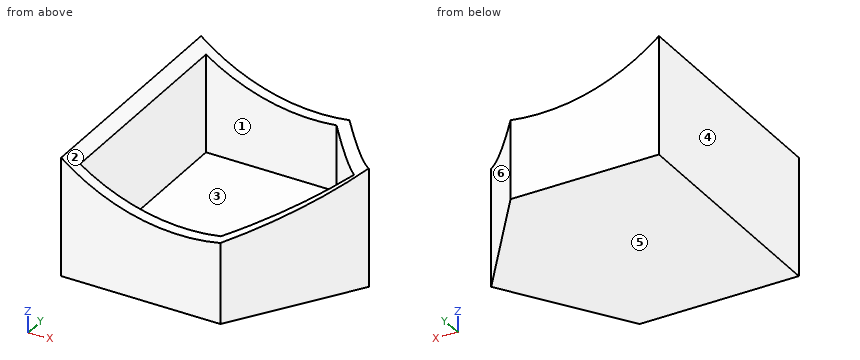
from build123d import *

# Parameters (mm, degrees)
F1_DEPTH = 50.8
F3_DEPTH = 46.571707
F4_T     = -2.54


with BuildPart() as f1:
    # F0 (on Front) → F1 (new body)
    with BuildSketch(Plane.XZ):
        with BuildLine():
            Line((-31.713647, -21.170707), (-31.713647, -46.570707))
            Line((-31.713647, -46.570707), (19.086353, -46.570707))
            Line((19.086353, -46.570707), (19.086353, -21.170707))
            ThreePointArc((19.086353, -21.170707), (-6.313647, -30.139476), (-31.713647, -21.170707))
        make_face()
    extrude(amount=F1_DEPTH)

    # F2 (on Top) → F3 (cut, through all)
    with BuildSketch(Plane.XY):
        Polygon((19.086353, -50.8), (19.086353, -25.4), (2.290366, -50.8), align=None)
        Polygon((19.086353, -25.4), (19.086353, 0), (0, 0), align=None)
    extrude(amount=-F3_DEPTH, mode=Mode.SUBTRACT)

    # F4
    f4_openings = [f1.faces().sort_by_distance(p)[0] for p in [
        (-6.313647, -25.4, -30.139476),
    ]]
    offset(amount=F4_T, openings=f4_openings)


solid = f1.part
Could you check a few things on this model? Use its own coordinates, in mm. Face numbers are marked on the shaded views. A direction names the side the tool comes from. Give positions to 0.01 mm unless a question says otherwise; leave off trailing zeros. Order: outer loops, then holes, each group sorted by start corner. A loop starts at its lowest first (then second) coordinate and runs counter-clockwise, first axis right, second up. Notation, with made-up numbers: (37.25, 88.5) - (56.25, 88.5) arc R15 ccw to (56.25, 108.5) - close; hole circle Ø7 at (14, 44.5). An arc over 180 degrees is marked (long way). One line per item, written item: value. Start each with the question number.
1. For P1, Ø10, axis at y = -31, z = -35.5, coming from the +X side; P2, Ø12, axis at x = -25.5, y = -9, coming from the +Z side; P3, Ø1.5, axis at x = -1.5, y = -38, coming from the +Z side, each with a flat end and sliding along its axis, tell me the tip position at first contact or that it passes through.
2. Imagine slicing it at D-D on y = -28.5. List the corners of the cut face in (x, z) for me.
3. Imagine slicing it at A-A on z = -32. List the corners of the cut face in (x, y) for me, plus the area to 3 significant figures.
4. Thinking about a two-plate mould opening in X: for the marked faces 3, 4, 5 and 6, which applies, +X half, -X half, draft (parallel to the pull), parting line (faces both ways), or undercut?
5. If I drill on probe 1 along Y at (x, z) = (-20, -38.5); probe 2 along Z at (x, y) = (-2, -3); probe 3 along X at (y, z) = (-39, -37.25), over which ranges is the centre line in solid material (lowest first)?
6. For the marked faces 1 and 2, which set-ups out of +Z, -Z, +X, -X, +Y, -Y let a thin tool reach every point of the face, with its end or its side?
7. Imagine slicing it at B-B on x = -27. List the corners of the cut face in (y, z) for me, plus the area to 3 significant figures.
8. Imagine slicing it at C-C on z = -26.5. List the corners of the cut face in (x, y) for me.
Values:
1. P1: x = 18.69
1. P2: z = -21.34
1. P3: z = -44.03
2. outline: (-31.71, -46.57) - (17.04, -46.57) - (17.04, -22.72) arc R40.45 cw to (13.99, -24.67) - (13.99, -44.03) - (-29.17, -44.03) - (-29.17, -23.06) arc R40.45 cw to (-31.71, -21.17) - close
3. outline: (-31.71, -50.8) - (2.29, -50.8) - (19.09, -25.4) - (0, 0) - (-31.71, 0) - close; hole (-29.17, -48.26) - (0.92, -48.26) - (15.98, -25.49) - (-1.27, -2.54) - (-29.17, -2.54) - close
3. area: 430 mm²
4. face 3: undercut
4. face 4: -X half
4. face 5: draft
4. face 6: +X half
5. probe 1: -50.8 to -48.26, -2.54 to 0
5. probe 2: -46.57 to -44.03
5. probe 3: -31.71 to -29.17, 7.05 to 10.09
6. face 1: +Z
6. face 2: +Z, +Y, -Y
7. outline: (-50.8, -46.57) - (0, -46.57) - (0, -24.45) - (-2.54, -24.45) - (-2.54, -44.03) - (-48.26, -44.03) - (-48.26, -24.45) - (-50.8, -24.45) - close
7. area: 229 mm²
8. outline: (-31.71, -50.8) - (-23.08, -50.8) - (-23.08, -48.26) - (-29.17, -48.26) - (-29.17, -2.54) - (-23.08, -2.54) - (-23.08, 0) - (-31.71, 0) - close; (10.46, -38.45) - (19.09, -25.4) - (10.46, -13.91) - (10.46, -18.14) - (15.98, -25.49) - (10.46, -33.85) - close
